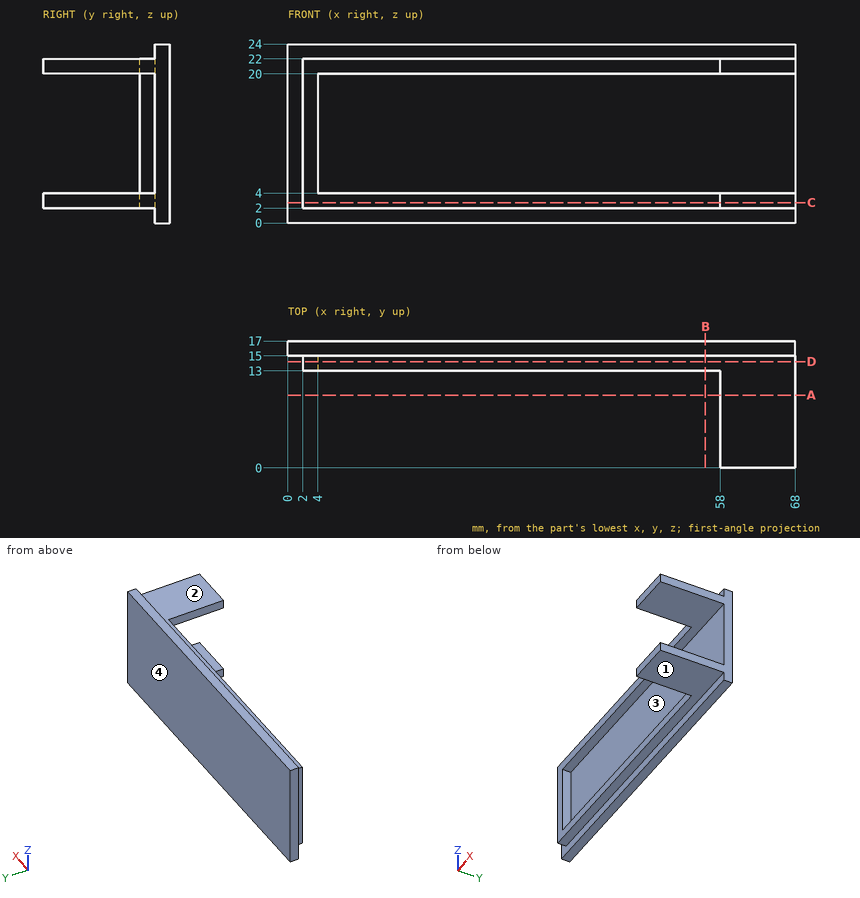
Could you check a few things on this drawing? It's one solid part, dimensions in mm from its lowest x, y, z. A direction names the side the tool comes from. Give positions to 0.01 mm unless a question says otherwise; leave off trailing zeros. Write each loop counter-clockwise with the first axis right and the second up, starting at its lowest first coordinate (ties: lowest second). Pieces come first, ordered by that corner, then holes. Notation, with made-up numbers: (-3.5, 14.5) -> (13.5, 14.5) arc R15 cw to (13.5, 39.5) -> close; hole circle Ø3 at (84.5, 84.5). An arc over 180 degrees is marked (long way). Answer as a JSON object with one key per item and string values.
Q1. Suppose I cut it at A-A on y = 9.75. Write out the boundary of the cut face in (x, z), then the cut area to 3 significant figures.
Taken from the geometry:
{"outline": "(58, 2) -> (68, 2) -> (68, 4) -> (58, 4) -> close; (58, 20) -> (68, 20) -> (68, 22) -> (58, 22) -> close", "area": "40.0 mm²"}
Q2. Will these pins go through, and if not, where does the flat tip stop? pin 1 Ø5 at (x, z) = (38, 9.5) entering from -Y; pin 2 Ø5 at (x, y) = (58.5, 3.5) entering from -Z; pin 3 Ø2 at (y, z) = (7.5, 20.5) entering from -X; pin 4 Ø2 at (y, z) = (5.5, 6.5) entering from -X.
Taken from the geometry:
{"pin 1": "stops at y = 15", "pin 2": "stops at z = 2", "pin 3": "stops at x = 58", "pin 4": "passes through"}
Q3. Suppose I cut it at C-C on z = 2.75. Write out the boundary of the cut face in (x, y).
Taken from the geometry:
{"outline": "(0, 15) -> (2, 15) -> (2, 13) -> (58, 13) -> (58, 0) -> (68, 0) -> (68, 17) -> (0, 17) -> close"}
Q4. Which directions (+Z, -Z, +X, -X, +Y, -Y) give clear straight access to the entire face, cutting with the end or side of a thin tool? Please do the marked faces 1, 2, 3 and 4.
Taken from the geometry:
{"face 1": "-Z, +X, -X, -Y", "face 2": "+Z, +X, -X, -Y", "face 3": "+X, -Y", "face 4": "+Z, -Z, +X, -X, +Y"}
Q5. Please list where these lines run through material, in increasing order: L1, parallel to Z at x = 61, y = 14.5; L2, parallel to Y at x = 8, z = 3.75; L3, parallel to Y at x = 39.5, z = 15.
Taken from the geometry:
{"L1": "z = 2 to 4, 20 to 22", "L2": "y = 13 to 17", "L3": "y = 15 to 17"}
Q6. Suppose I cut it at B-B on x = 56. Write out the boundary of the cut face in (y, z), then the cut area to 3 significant figures.
Taken from the geometry:
{"outline": "(13, 2) -> (15, 2) -> (15, 0) -> (17, 0) -> (17, 24) -> (15, 24) -> (15, 22) -> (13, 22) -> (13, 20) -> (15, 20) -> (15, 4) -> (13, 4) -> close", "area": "56.0 mm²"}
Q7. Suppose I cut it at D-D on y = 14.25. Write out the boundary of the cut face in (x, z).
Taken from the geometry:
{"outline": "(2, 2) -> (68, 2) -> (68, 4) -> (4, 4) -> (4, 20) -> (68, 20) -> (68, 22) -> (2, 22) -> close"}
